Geometry check sheet. Reference: the model listing, model coordinates, mm. Face numbers are marked on the shaded views. A direction names the side the tool comes from. Coordinates: 2 decimals unless noted, no trailing zeros. Order: outer loops, then holes, each group sorted by start corner. A loop starts at its lowest first (then second) coordinate and runs counter-clockwise, first axis right, second up. Notation, with made-up numbers: (70, 75.25) - (106, 75.25) arc R12 ccw to (106, 82.25) - close; hole circle Ø10 at (88, -14). An arc over 180 degrees is marked (long way). Use CSV: the item, a comma, the result in double quotes. Start each with the question number.
1) Thickness scan on probe 1 along Y at (x, z) = (-35, 4.5); probe 2 along X at (y, z) = (-35.5, 10); probe 3 along Y at (x, z) = (0, 6.5). Record the ranges inside material, lowest first. Write a range as [from, to].
2) Tool access check on the marked faces 5, 6, 7 and 8. Record the directions out of +Z, -Z, +X, -X, +Y, -Y that give a thin tool (end or side, any length) a straight path to the whole face; none if there is none.
3) Sectioned sample at D-D, the plane y = 7. Record the cut outline in (x, z), and give its area (3 significant figures).
4) Sectioned sample at B-B, the plane y = -35. Record the cut outline in (x, z).
5) Depth check by flat-ended pin: P1, Ø15.5, axis at x = -35, y = -35, coming from the -Z side; P2, Ø8, axis at y = 8, z = 7.5, coming from the -X side; P3, Ø8, axis at y = 0.5, z = 6.5, coming from the +X side. Enter the tip coordinate at first touch or a pass-through.
6) Sectioned sample at A-A, the plane x = 35. Record the cut outline in (y, z), and give its area (3 significant figures).
7) Sectioned sample at C-C, the plane z = 8.75. Record the cut outline in (x, y), and give its area (3 significant figures).
8) Draft check along X on the marked faces 1, 2, 3 and 4. Enter one of: released by +X, released by -X, zero draft, split by the parting line, or undercut.
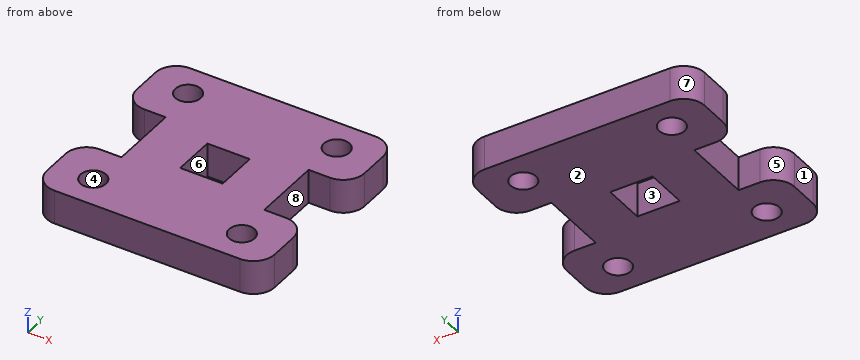
from build123d import *

# Parameters (mm, degrees)
F0_R     = 6
F1_DEPTH = 16


with BuildPart() as f1:
    # F0 (on Top) → F1 (new body)
    with BuildSketch(Plane.XY):
        with BuildLine():
            Line((-33.65, 3.65), (-33.65, -3.65))
            Line((-33.65, -3.65), (-33.65, -16.35))
            Line((-33.65, -16.35), (-43.65, -16.35))
            ThreePointArc((-43.65, -16.35), (-50.721068, -19.278932), (-53.65, -26.35))
            Line((-53.65, -26.35), (-53.65, -40))
            ThreePointArc((-53.65, -40), (-50.721068, -47.071068), (-43.65, -50))
            Line((-43.65, -50), (0, -50))
            Line((0, -50), (43.65, -50))
            ThreePointArc((43.65, -50), (50.721068, -47.071068), (53.65, -40))
            Line((53.65, -40), (53.65, -26.35))
            ThreePointArc((53.65, -26.35), (50.721068, -19.278932), (43.65, -16.35))
            Line((43.65, -16.35), (33.65, -16.35))
            Line((33.65, -16.35), (33.65, -3.65))
            Line((33.65, -3.65), (33.65, 3.65))
            Line((33.65, 3.65), (33.65, 16.35))
            Line((33.65, 16.35), (43.65, 16.35))
            ThreePointArc((43.65, 16.35), (50.721068, 19.278932), (53.65, 26.35))
            Line((53.65, 26.35), (53.65, 40))
            ThreePointArc((53.65, 40), (50.721068, 47.071068), (43.65, 50))
            Line((43.65, 50), (0, 50))
            Line((0, 50), (-43.65, 50))
            ThreePointArc((-43.65, 50), (-50.721068, 47.071068), (-53.65, 40))
            Line((-53.65, 40), (-53.65, 26.35))
            ThreePointArc((-53.65, 26.35), (-50.721068, 19.278932), (-43.65, 16.35))
            Line((-43.65, 16.35), (-33.65, 16.35))
            Line((-33.65, 16.35), (-33.65, 3.65))
        make_face()
        with Locations((-35, -35)):
            Circle(F0_R, mode=Mode.SUBTRACT)
        with Locations((35, -35)):
            Circle(F0_R, mode=Mode.SUBTRACT)
        with Locations((-35, 35)):
            Circle(F0_R, mode=Mode.SUBTRACT)
        Polygon((-10, -10), (-10, 0), (-10, 10), (0, 10), (10, 10), (10, 0), (10, -10), (0, -10), align=None, mode=Mode.SUBTRACT)
        with Locations((35, 35)):
            Circle(F0_R, mode=Mode.SUBTRACT)
    extrude(amount=F1_DEPTH)


solid = f1.part
Evaluation:
1,probe 1,"[-50, -41], [-29, -16.35], [16.35, 29], [41, 50]"
1,probe 2,"[-53.65, -40.98], [-29.02, 29.02], [40.98, 53.65]"
1,probe 3,"[-50, -10], [10, 50]"
2,face 5,"+Z, -Z, -X"
2,face 6,"+Z, -Z"
2,face 7,"+Z, -Z, -X, +Y"
2,face 8,"+Z, -Z, +X"
3,outline,"(-33.65, 0) - (-10, 0) - (-10, 16) - (-33.65, 16) - close; (10, 0) - (33.65, 0) - (33.65, 16) - (10, 16) - close"
3,area,"757 mm²"
4,outline,"(-53.65, 0) - (-41, 0) - (-41, 16) - (-53.65, 16) - close; (-29, 0) - (29, 0) - (29, 16) - (-29, 16) - close; (41, 0) - (53.65, 0) - (53.65, 16) - (41, 16) - close"
5,P1,"z = 0"
5,P2,"x = -33.65"
5,P3,"x = 33.65"
6,outline,"(-50, 0) - (-41, 0) - (-41, 16) - (-50, 16) - close; (-29, 0) - (-16.35, 0) - (-16.35, 16) - (-29, 16) - close; (16.35, 0) - (29, 0) - (29, 16) - (16.35, 16) - close; (41, 0) - (50, 0) - (50, 16) - (41, 16) - close"
6,area,"693 mm²"
7,outline,"(-53.65, -40) arc R10 ccw to (-43.65, -50) - (43.65, -50) arc R10 ccw to (53.65, -40) - (53.65, -26.35) arc R10 ccw to (43.65, -16.35) - (33.65, -16.35) - (33.65, 16.35) - (43.65, 16.35) arc R10 ccw to (53.65, 26.35) - (53.65, 40) arc R10 ccw to (43.65, 50) - (-43.65, 50) arc R10 ccw to (-53.65, 40) - (-53.65, 26.35) arc R10 ccw to (-43.65, 16.35) - (-33.65, 16.35) - (-33.65, -16.35) - (-43.65, -16.35) arc R10 ccw to (-53.65, -26.35) - close; hole circle Ø12 at (-35, -35); hole circle Ø12 at (-35, 35); hole (-10, -10) - (10, -10) - (10, 10) - (-10, 10) - close; hole circle Ø12 at (35, -35); hole circle Ø12 at (35, 35)"
7,area,"8,400 mm²"
8,face 1,"released by -X"
8,face 2,"zero draft"
8,face 3,"undercut"
8,face 4,"undercut"
